Part model, mm, in its own coordinate system. A direction names the side the tool comes from. Coordinates: 2 decimals unless noted, no trailing zeros. Write each loop counter-clockwise with the first axis right and the second up, starting at its lowest first coordinate (ties: lowest second). Pieces come first, ordered by that corner, then holes. Notation, with made-up numbers: M -36,49.5 L -30,49.5 A27 cw -30,66.5 Z; hole C 65.25,65.25 d7. An arc over 180 degrees is marked long. Use a Markdown table: item, result. Add a question column.
Q1. Slice it at A-A on y = 0.75. Write the cut outline in (x, z).
Q2. Slice it at C-C on z = 2.5. Write the cut outline in (x, y), then the cut area to 3 significant figures.
Q3. Slice it at B-B on y = 10. Write the cut outline in (x, z), then the cut area to 3 significant figures.
Q4. Mould opens along X. For faces 3 (the cylindrical face through (6.859, 6.797, 1.479)), 4 (the cylindrical face through (12.297, -13.859, 1.521)), 5 (the flat face through (-13.5, 0, 1)) say: released by +X, released by -X, zero draft, split by the parting line, or undercut.
Q5. Slice it at D-D on x = 2.5. Write the cut outline in (y, z), then the cut area to 3 significant figures.
Q6. Wall check: L1, parallel to Y at x = -0.5, z = 1.85; L2, parallel to Y at x = 10.5, z = 1.7; L3, parallel to Y at x = -10, z = 1.35. Give the ranges that are in metal, low to high. Write a range as from..to.
Q7. Tool access for faces 1 (the cylindrical face through (-6.797, 6.859, 1.479)), 2 (the flat face through (13.5, 0, 1)): list every direction of +Z, -Z, +X, -X, +Y, -Y with a clear straight run to the whole face (end or side of a thin tool).
from build123d import *

# Parameters (mm, degrees)
SKETCH_1_W          = 27
SKETCH_1_H          = 30
SKETCH_1_R          = 1.6
EXTRUDE_1_DEPTH     = 3
SKETCH_2_W          = 16
SKETCH_2_H          = 16
CUT_EXTRUDE_1_DEPTH = 4
FILLET_1_R          = 4


with BuildPart() as part:
    # 草图1 → 凸台-拉伸1 (new body)
    with BuildSketch(Plane.XY):
        Rectangle(SKETCH_1_W, SKETCH_1_H)
        with Locations((10, 10)):
            Circle(SKETCH_1_R, mode=Mode.SUBTRACT)
        with Locations((10, -10)):
            Circle(SKETCH_1_R, mode=Mode.SUBTRACT)
        with Locations((-10, -10)):
            Circle(SKETCH_1_R, mode=Mode.SUBTRACT)
        with Locations((-10, 10)):
            Circle(SKETCH_1_R, mode=Mode.SUBTRACT)
    extrude(amount=EXTRUDE_1_DEPTH)

    # 草图2 → 切除-拉伸1 (cut, through all)
    with BuildSketch(Plane.XY.offset(3)):
        Rectangle(SKETCH_2_W, SKETCH_2_H)
    extrude(amount=-CUT_EXTRUDE_1_DEPTH, mode=Mode.SUBTRACT)

    # 圆角1
    fillet_1_edges = [part.edges().sort_by_distance(p)[0] for p in [
        (8, 8, 1.5),
        (8, -8, 1.5),
        (-8, -8, 1.5),
        (-8, 8, 1.5),
        (13.5, -15, 1.5),
        (-13.5, -15, 1.5),
        (-13.5, 15, 1.5),
        (13.5, 15, 1.5),
    ]]
    fillet(fillet_1_edges, radius=FILLET_1_R)


solid = part.part
Recorded:
| question | item | result |
|---|---|---|
| 1 | outline | M -13.5,0 L -8,0 L -8,3 L -13.5,3 Z; M 8,0 L 13.5,0 L 13.5,3 L 8,3 Z |
| 2 | outline | M -13.5,-11 A4 ccw -9.5,-15 L 9.5,-15 A4 ccw 13.5,-11 L 13.5,11 A4 ccw 9.5,15 L -9.5,15 A4 ccw -13.5,11 Z; hole C -10,-10 d3.2; hole C -10,10 d3.2; hole M -8,-4 A4 ccw -4,-8 L 4,-8 A4 ccw 8,-4 L 8,4 A4 ccw 4,8 L -4,8 A4 ccw -8,4 Z; hole C 10,-10 d3.2; hole C 10,10 d3.2 |
| 2 | area | 522 mm² |
| 3 | outline | M -13.5,0 L -11.6,0 L -11.6,3 L -13.5,3 Z; M -8.4,0 L 8.4,0 L 8.4,3 L -8.4,3 Z; M 11.6,0 L 13.5,0 L 13.5,3 L 11.6,3 Z |
| 3 | area | 61.8 mm² |
| 4 | face 3 | undercut |
| 4 | face 4 | released by +X |
| 4 | face 5 | released by -X |
| 5 | outline | M -15,0 L -8,0 L -8,3 L -15,3 Z; M 8,0 L 15,0 L 15,3 L 8,3 Z |
| 5 | area | 42.0 mm² |
| 6 | L1 | -15..-8, 8..15 |
| 6 | L2 | -14.87..-11.52, -8.48..8.48, 11.52..14.87 |
| 6 | L3 | -14.97..-11.6, -8.4..8.4, 11.6..14.97 |
| 7 | face 1 | +Z, -Z |
| 7 | face 2 | +Z, -Z, +X, +Y, -Y |
